The drawing under review shows one solid part. Ordinate dimensions are in mm from its lowest x, y, z. Give positions to 0.01 mm unless a question says otherwise; leave off trailing zeros. Loops run counter-clockwise (first coordinate to the right, second up) from the corner with the lowest first, then second, coordinate; pieces in that order, holes last. Notation, with made-up numbers: M 12.5,6 L 71.5,6 A17 cw 71.5,37 Z; hole C -24,49.25 d5. An arc over 180 degrees is marked long. Answer as CSV lines item,"result".
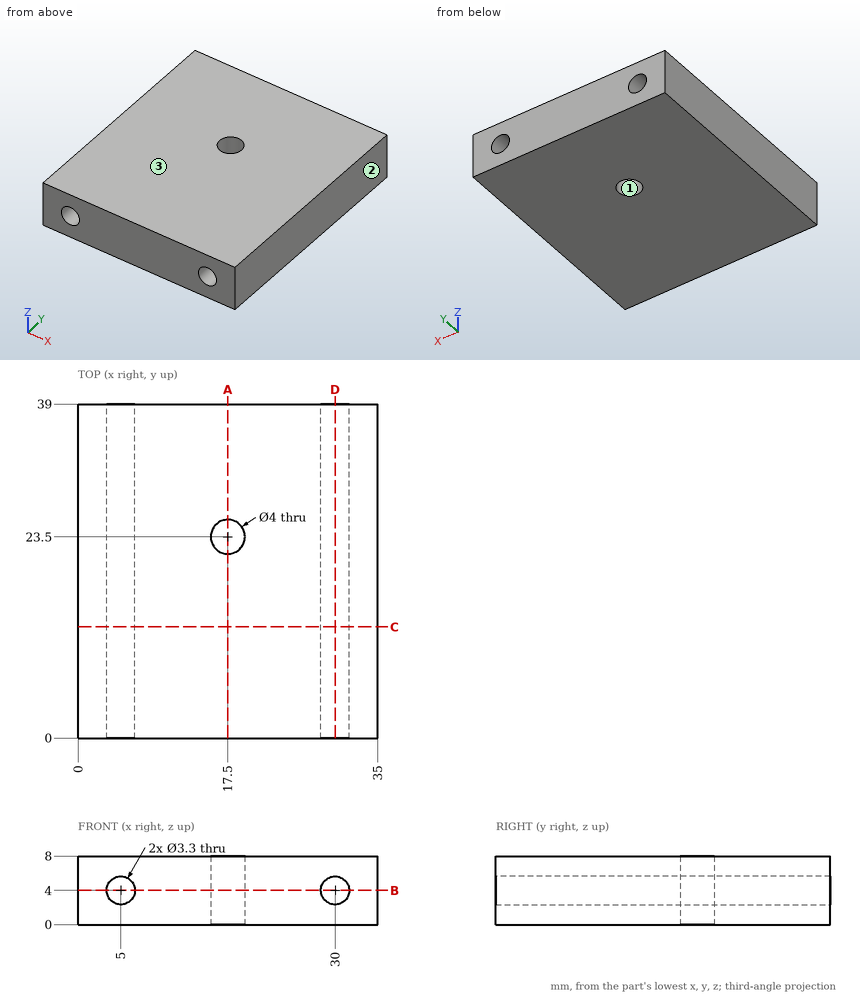
1. We need section D-D, the plane x = 30. Write out the cut boundary in (y, z).
Answer block:
outline,"M 0,0 L 39,0 L 39,2.35 L 0,2.35 Z; M 0,5.65 L 39,5.65 L 39,8 L 0,8 Z"
2. To check wall thickness, follow L1, parallel to X at y = 10, z = 4; L2, parallel to Y at x = 17.5, z = 6.25; L3, parallel to X at y = 34, z = 2.5. State the ranges of each line that lie inside material, in increasing order. Write a range as [from, to].
Answer block:
L1,"[0, 3.35], [6.65, 28.35], [31.65, 35]"
L2,"[0, 21.5], [25.5, 39]"
L3,"[0, 4.31], [5.69, 29.31], [30.69, 35]"
3. We need section B-B, the plane z = 4. Write out the cut boundary in (x, y).
Answer block:
outline,"M 0,0 L 3.35,0 L 3.35,39 L 0,39 Z; M 6.65,0 L 28.35,0 L 28.35,39 L 6.65,39 Z; M 31.65,0 L 35,0 L 35,39 L 31.65,39 Z; hole C 17.5,23.5 d4"
4. We need section C-C, the plane y = 13. Write out the cut boundary in (x, z), plus the area to 3 significant figures.
Answer block:
outline,"M 0,0 L 35,0 L 35,8 L 0,8 Z; hole C 5,4 d3.3; hole C 30,4 d3.3"
area,"263 mm²"
5. We need section A-A, the plane x = 17.5. Write out the cut boundary in (y, z).
Answer block:
outline,"M 0,0 L 21.5,0 L 21.5,8 L 0,8 Z; M 25.5,0 L 39,0 L 39,8 L 25.5,8 Z"
6. The part is to be moulded in two halves that separate along X. For the marked faces 1, 2 and 3, say which applies: pulls with the +X half, pulls with the -X half, needs draft (parallel to the pull), parting line crosses it, or undercut.
Answer block:
face 1,"undercut"
face 2,"pulls with the +X half"
face 3,"needs draft"
